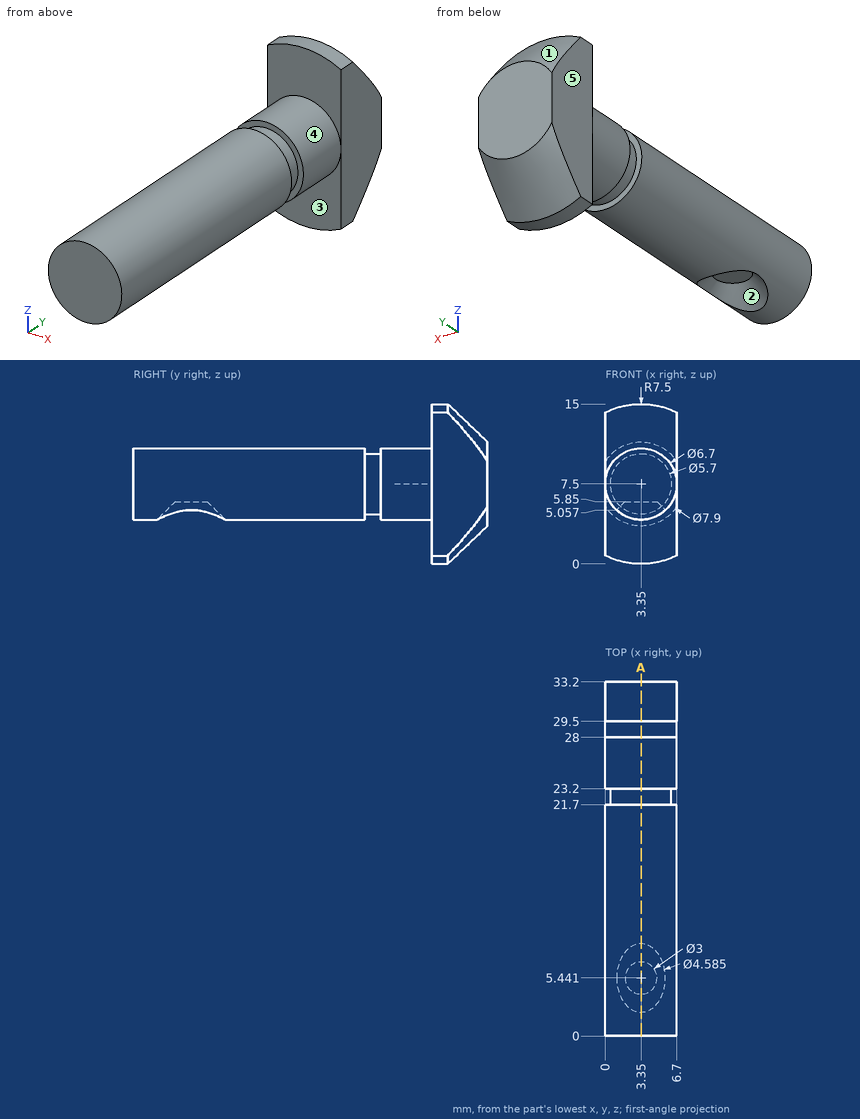
Design review of the part shown in the three views and the two pictorial views. Dimensions are in mm from the part's minimum x, y and z. A direction names the side the tool comes from. Give positions to 0.01 mm unless a question says otherwise; leave off trailing zeros. Loops run counter-clockwise (first coordinate to the right, second up) from the corner with the lowest first, then second, coordinate; pieces in that order, holes last. Notation, with made-up numbers: (45.5, 28.25) -> (93.5, 28.25) arc R7 cw to (93.5, 38.25) -> close; hole circle Ø2 at (61, -38). An arc over 180 degrees is marked (long way). Put each result on its own line as item: value. Start each with the question number.
1. Mouldability with a two-part tool opening along X and no side actions: class the marked faces 1, 2 and 3 as released by +X, released by -X, zero draft, split by the parting line, or undercut.
2. Clearance check with flat-ended pins moving along their axes: P1, Ø6, axis at y = 9, z = 12.5, coming from the -X side; P2, Ø1, axis at x = 4.5, y = 15.5, coming from the -Z side; P3, Ø1.5, axis at x = 1.5, y = 15.5, coming from the +Z side (1 decimal). State where each tip first meets the part, or that it passes through.
3. Wall thickness on probe 1 along X at (y, z) = (24, 9.25) (1 decimal); probe 2 along Z at (x, y) = (3.5, 5); probe 3 along Z at (x, y) = (0.5, 5.5): over which ranges is each line inside the solid? List them lowest first.
4. We need section A-A on x = 3.35. State the section outline as (y, z) points, then the cut area to 3 significant figures.
5. For the marked faces 4 and 5, list the 3-axis set-ups (+Z, -Z, +X, -X, +Y, -Y) from which the entire face can be reached by the end or side of a thin tool; tool diameter is ignored.
Determined:
1. face 1: split by the parting line
1. face 2: undercut
1. face 3: zero draft
2. P1: x = 0.66
2. P2: z = 4.21
2. P3: z = 10.7
3. probe 1: 0.5 to 6.2
3. probe 2: 5.85 to 10.85
3. probe 3: 5.74 to 9.26
4. outline: (0, 4.15) -> (2.24, 4.15) -> (3.94, 5.85) -> (6.94, 5.85) -> (8.64, 4.15) -> (21.7, 4.15) -> (21.7, 4.65) -> (23.2, 4.65) -> (23.2, 4.15) -> (28, 4.15) -> (28, 0) -> (29.5, 0) -> (33.2, 3.55) -> (33.2, 11.45) -> (29.5, 15) -> (28, 15) -> (28, 10.85) -> (23.2, 10.85) -> (23.2, 10.35) -> (21.7, 10.35) -> (21.7, 10.85) -> (0, 10.85) -> close
4. area: 243 mm^2
5. face 4: -Y
5. face 5: +Z, -Z, -X, +Y, -Y
